The drawing under review shows one solid part. Ordinate dimensions are in mm from its lowest x, y, z. Coordinates: 2 decimals unless noted, no trailing zeros. Order: outer loops, then holes, each group sorted by start corner. A loop starts at its lowest first (then second) coordinate and runs counter-clockwise, first axis right, second up.
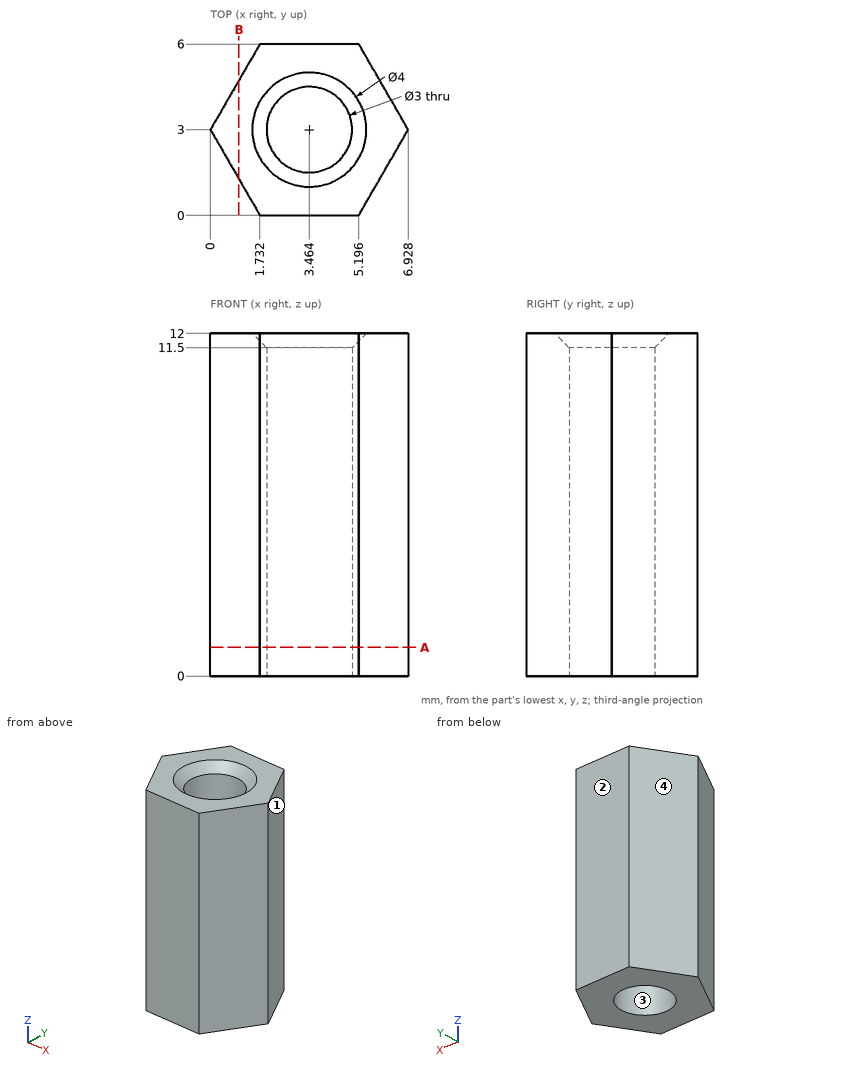
(1) For pin 1 Ø2 at (y, z) = (1, 5) entering from -X, flat-tipped, find the tip position at first contact; note if it passes through.
A:
pin 1: stops at x = 0.58
(2) We need section B-B, the plane x = 1. Write out the cut boundary in (y, z).
A:
outline: (1.27, 0) - (4.73, 0) - (4.73, 12) - (1.27, 12) - close
(3) Draft analysis for pull direction X (two halves, no side actions). For the marked faces 1, 2, 3 and 4, state which applies: released by +X, released by -X, zero draft, split by the parting line, or undercut.
A:
face 1: released by +X
face 2: zero draft
face 3: undercut
face 4: released by -X
(4) We need section A-A, the plane z = 1. Write out the cut boundary in (x, y).
A:
outline: (0, 3) - (1.73, 0) - (5.2, 0) - (6.93, 3) - (5.2, 6) - (1.73, 6) - close; hole circle Ø3 at (3.46, 3)
(5) Wall thickness on probe 1 along X at (y, z) = (3.75, 9) (1 decimal); probe 2 along Y at (x, z) = (4.75, 5.5); probe 3 along Y at (x, z) = (4, 2): over which ranges is each line inside the solid? List them lowest first.
A:
probe 1: x = 0.4 to 2.2, 4.8 to 6.5
probe 2: y = 0 to 2.23, 3.77 to 6
probe 3: y = 0 to 1.6, 4.4 to 6
